Work out the finished part from the listing and answer in its coordinate system (mm). A direction names the side the tool comes from. Coordinates: 2 decimals unless noted, no trailing zeros. Write each loop counter-clockwise with the first axis right and the second up, starting at its lowest first coordinate (ties: lowest second). Pieces come first, ordered by that corner, then holes. Notation, with made-up numbers: (68.5, 77.5) - (102.5, 77.5) arc R21 cw to (102.5, 86.5) - close; hole circle Ø3 at (80.5, 21.5). An arc over 180 degrees is marked (long way). One line per item, written item: value.
Autodesk Inventor part; units mm, degrees
ref_plane "YZ Plane" through (0, 0, 0) normal (1, 0, 0) x (0, 1, 0)
ref_plane "XZ Plane" through (0, 0, 0) normal (0, 1, 0) x (-1, 0, 0)
ref_plane "XY Plane" through (0, 0, 0) normal (0, 0, 1) x (1, 0, 0)
sketch "Sketch1" plane through (0, 0, 0) normal (1, 0, 0) x (0, 1, 0)
  line L0 (9, 10) -> (-9, 10)
  line L1 (-9, 10) -> (-9, -10)
  line L2 (-9, -10) -> (9, -10)
  line L3 (9, -10) -> (9, 10)
  line L4 (9, 10) -> (-9, -10) construction
  line L5 (-9, 10) -> (9, -10) construction
  line L6 (-11, 12) -> (11, 12)
  line L7 (11, 12) -> (11, -12)
  line L8 (11, -12) -> (-11, -12)
  line L9 (-11, -12) -> (-11, 12)
  line L10 (-11, 12) -> (9, 32)
  line L11 (-11, 12) -> (21.2472, 12) construction
  line L12 (11, 12) -> (11, 32)
  line L13 (-11, -12) -> (9, -32)
  line L14 (-11, -12) -> (29.5291, -12) construction
  line L15 (11, -12) -> (11, -32)
  line L16 (9, 12) -> (9, 29.1716)
  line L17 (9, 29.1716) -> (-8.1716, 12)
  line L18 (-8.1716, -12) -> (9, -29.1716)
  line L19 (9, -29.1716) -> (9, -12)
  line L20 (11, 12) -> (11, 10)
  line L21 (11, 12) -> (9, 12)
  line L22 (-8.1716, 12) -> (-11, 12)
  line L23 (-11, -12) -> (-8.1716, -12)
  line L24 (11, -12) -> (9, -12)
  line L25 (9, 29.1716) -> (9, 32)
  line L26 (9, 32) -> (11, 32)
  line L27 (9, -29.1716) -> (11, -29.1716)
  line L28 (9, -29.1716) -> (9, -32)
  line L29 (9, -32) -> (11, -32)
  line L30 (11, 12) -> (9, 12)
  line L31 (-8.1716, 12) -> (-11, 12)
  line L32 (-8.1716, 12) -> (9, 29.1716)
  line L33 (-8.1716, -12) -> (9, -12)
  line L34 (11, -12) -> (9, -12)
  point P0 (0, 0)
  dimension "d0" = 18
  dimension "d1" = 20
  dimension "d2" = 2
  dimension "d3" = 45
  dimension "d4" = 45
  dimension "d5" = 2
  dimension "d6" = 2
extrude "Extrusion2" add sketch "Sketch1" along normal blind 15 contours L10 L25 L17 L6 | L6 L7 L8 L9 | L8 L18 L28 L13 | L26 L12 L6 L16 L25 | L28 L27 L15 L29 | L8 L15 L27 L19
properties part number "Motor_Shroud"
Item 1: Section D-D, the plane z = 28 is taken. Determine the outline of the cut face in (x, y), then the cut area to 3 significant figures.
Evaluation:
outline: (0, 5) - (15, 5) - (15, 7.83) - (0, 7.83) - close; (0, 9) - (15, 9) - (15, 11) - (0, 11) - close
area: 72.4 mm2
Item 2: Consider probe 1 along Y at (x, z) = (6.75, 9); probe 2 along Z at (x, y) = (11, -8); probe 3 along Z at (x, y) = (12.5, 6.5). Determine where each line is inside the solid, lowest interval first.
Evaluation:
probe 1: y = -11 to -9, 9 to 11
probe 2: z = -15 to -12.17, -12 to -10, 10 to 12, 12.17 to 15
probe 3: z = -29.5 to -26.67, -12 to -10, 10 to 12, 26.67 to 29.5
Item 3: Which of the six approach directions +Z, -Z, +X, -X, +Y, -Y give full straight-line access (tool end or side, diameter ignored) to faces 1 (the face through (7, 11, 0)), 2 (the face through (7, 0, 10))?
Evaluation:
face 1: +Z, -Z, +X, -X, +Y
face 2: +X, -X
Item 4: Section C-C, the plane y = -3 is taken. Determine the outline of the cut face in (x, z), then the cut area to 3 significant figures.
Evaluation:
outline: (0, -20) - (15, -20) - (15, -17.17) - (0, -17.17) - close; (0, -12) - (15, -12) - (15, -10) - (0, -10) - close; (0, 10) - (15, 10) - (15, 12) - (0, 12) - close; (0, 17.17) - (15, 17.17) - (15, 20) - (0, 20) - close
area: 145 mm2
Item 5: Section A-A, the plane z = -9 is taken. Determine the outline of the cut face in (x, y), then the cut area to 3 significant figures.
Evaluation:
outline: (0, -11) - (15, -11) - (15, -9) - (0, -9) - close; (0, 9) - (15, 9) - (15, 11) - (0, 11) - close
area: 60.0 mm2
Item 6: Determine the mould class of faces 3 (the face through (7, -1, 22)), 4 (the face through (7, 9, 20)), 5 (the face through (7, -11, 0)) for opening direction Z: +Z half, -Z half, draft (parallel to the pull), parting line (faces both ways), or undercut.
Evaluation:
face 3: +Z half
face 4: undercut
face 5: draft
Item 7: Given pin 1 (4.5 mm diameter, centred on x = 7, z = 20, fed in from -Y); pin 2 (1.5 mm diameter, centred on x = 13, y = -6.5, fed in from +Z); pin 3 (6 mm diameter, centred on x = 11.5, y = -1, fed in from -Z); pin 4 (5 mm diameter, centred on y = -3.5, z = 25.5, fed in from +X), each flat-ended and moving along its own axis, determine where each tip first touches the part or whether it passes through.
Evaluation:
pin 1: stops at y = -5.25
pin 2: stops at z = 17.25
pin 3: stops at z = -25
pin 4: passes through
Item 8: Section B-B, the plane x = 1.25 is taken. Determine the outline of the cut face in (y, z).
Evaluation:
outline: (-11, -12) - (9, -32) - (11, -32) - (11, 32) - (9, 32) - (-11, 12) - close; hole (-9, -10) - (9, -10) - (9, 10) - (-9, 10) - close; hole (-8.17, -12) - (9, -29.17) - (9, -12) - close; hole (-8.17, 12) - (9, 12) - (9, 29.17) - close
